```python
from build123d import *

# Parameters (mm, degrees)
SKETCH2_W           = 16.351115912
SKETCH2_H           = 2.286251171
CUT_EXTRUDE2_DEPTH  = 8
CIRPATTERN1_COUNT   = 10
BOSS_EXTRUDE2_DEPTH = 23
CIRPATTERN2_COUNT   = 3


with BuildPart() as part:
    # Sketch1 → Revolve1 (revolve)
    with BuildSketch(Plane.XY):
        Polygon((-45, 22.5), (-20, 22.5), (-20, 17.8), (4, 17.8), (4, 7.8), (-59, 7.8), (-59, 13), (-84, 13), (-84, 14.303183025), (-75, 19.499335448), (-45, 24.089980537), align=None)
    revolve(axis=Axis((-59, 7.8, 0), (1, 0, 0)))

    # Sketch2 → Cut-Extrude2 (cut)
    with BuildSketch(Plane(origin=(0, 0, 0), x_dir=(1, 0, 0), z_dir=(0, 1, 0))):
        with Locations((-60.455240296, 1.143125585)):
            Rectangle(SKETCH2_W, SKETCH2_H)
    cut_extrude2 = extrude(amount=-CUT_EXTRUDE2_DEPTH, mode=Mode.SUBTRACT)

    # CirPattern1: Cut-Extrude2 ×10 about axis
    cirpattern1_axis = Axis((0, 7.8, 0), (1, 0, 0))
    for i in range(1, CIRPATTERN1_COUNT):
        add(cut_extrude2.rotate(cirpattern1_axis, i * 360 / CIRPATTERN1_COUNT), mode=Mode.SUBTRACT)

    # Sketch3 → Boss-Extrude2 (add)
    with BuildSketch(Plane.ZY.offset(59)):
        with BuildLine():
            ThreePointArc((2.388609227, 12.418933423), (0.326387029, 12.989746767), (-1.791101139, 12.681798512))
            Line((-1.791101139, 12.681798512), (-0.861106317, 10.147018515))
            ThreePointArc((-0.861106317, 10.147018515), (0.156916841, 10.295070561), (1.148369821, 10.020641069))
            Line((1.148369821, 10.020641069), (2.388609227, 12.418933423))
        make_face()
    boss_extrude2 = extrude(amount=BOSS_EXTRUDE2_DEPTH)

    # CirPattern2: Boss-Extrude2 ×3 about axis
    cirpattern2_axis = Axis((0, 7.8, 0), (1, 0, 0))
    for i in range(1, CIRPATTERN2_COUNT):
        add(boss_extrude2.rotate(cirpattern2_axis, i * 360 / CIRPATTERN2_COUNT))


solid = part.part
```
Could you check a few things on this model? Use its own coordinates, in mm. A direction names the side the tool comes from. Round coordinates to 2 decimals unless told otherwise and drop trailing zeros. Loops run counter-clockwise (first coordinate to the right, second up) from the corner with the lowest first, then second, coordinate; pieces in that order, holes last. Notation, with made-up numbers: (-32.75, 82.25) - (13.25, 82.25) arc R36 ccw to (13.25, 121.25) - close; hole circle Ø8 at (35, 3.5). An arc over 180 degrees is marked (long way). Answer in a Markdown table with one row per item. Add a question column.
(1) If we section it at A-A (x = -76): Please give me the cut outline in (y, z), plus the area to 3 significant figures.
(2) If we section it at C-C (x = -50): Please give me the cut outline in (y, z), plus the area to 3 significant figures.
(3) For faces 1 (the face through (-70.34, 4.57, 2.07)), 2 (the face through (-60.57, 16.39, 6.24)), 3 (the face through (-52.28, -4, -1)), which set-ups out of +Z, -Z, +X, -X, +Y, -Y let a thin tool reach every point of the face, with its end or its side?
(4) If we section it at B-B (x = -28): Please give me the cut outline in (y, z), plus the area to 3 significant figures.
(5) I'm going to push flat-ended pins straight in: pin 1 (5 mm diameter, centred on x = -54, y = 10.5, fed in from -Z); pin 2 (1.5 mm diameter, centred on x = -7, y = 1.5, fed in from -Z); pin 3 (1.8 mm diameter, centred on x = -59.5, z = -1.5, fed in from -Y). Where does each tip first touch, or does it pass through?
(6) If we mould it in two halves opening along Y, with no side actions, what happens to faces 4 (the face through (-61, -3, -2.286)), 5 (the face through (-60.57, 6.714, -10.741))? For each: pulls with the +Y half, pulls with the -Y half, needs draft (parallel to the pull), parting line crosses it, or undercut.
(7) I need wall thicknesses on line 1 along X through (y, z) = (-7, -1); line 2 along Y through (x, z) = (-54, -6); line 3 along Z through (x, y) = (-63, 0.5). Which ranges of each line are inside material? Lowest first, please.
Model answer:
| question | item | result |
|---|---|---|
| 1 | outline | circle Ø22.24 at (7.8, 0); hole (3.42, 2.81) arc R5.2 ccw to (3.81, -3.33) - (5.88, -1.6) arc R2.5 ccw to (7.68, -2.5) - (7.56, -5.19) arc R5.2 ccw to (12.68, -1.79) - (10.15, -0.86) arc R2.5 ccw to (10.02, 1.15) - (12.42, 2.39) arc R5.2 ccw to (6.91, 5.12) - (7.37, 2.46) arc R2.5 ccw to (5.7, 1.35) - close |
| 1 | area | 330 mm² |
| 2 | outline | circle Ø31.05 at (7.8, 0) |
| 2 | area | 757 mm² |
| 3 | face 1 | -X |
| 3 | face 2 | none |
| 3 | face 3 | -Y |
| 4 | outline | circle Ø29.4 at (7.8, 0) |
| 4 | area | 679 mm² |
| 5 | pin 1 | stops at z = -15.18 |
| 5 | pin 2 | stops at z = -8.32 |
| 5 | pin 3 | stops at y = -6.15 |
| 6 | face 4 | needs draft |
| 6 | face 5 | undercut |
| 7 | line 1 | x = -52.28 to -45 |
| 7 | line 2 | y = -5.85 to -0.46, 2.52 to 16.06, 19.95 to 21.45 |
| 7 | line 3 | z = -11.4 to -8.13, -5.3 to 3.22, 5.3 to 11.4 |
